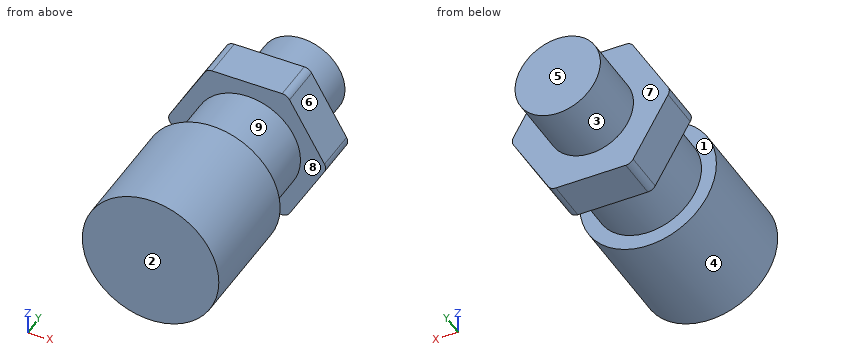
from build123d import *

# Parameters (mm, degrees)
BOSS_EXTRUDE1_DEPTH = 12.7
FILLET1_R           = 2.54
SKETCH2_R           = 20.32
BOSS_EXTRUDE4_DEPTH = 55.626
SKETCH4_R           = 20.32
SKETCH4_R_2         = 15.875
CUT_EXTRUDE1_DEPTH  = 20.32
SKETCH5_R           = 12.7
BOSS_EXTRUDE5_DEPTH = 19.05


with BuildPart() as part:
    # Sketch1 → Boss-Extrude1 (new body)
    with BuildSketch(Plane(origin=(0, 0, 0), x_dir=(1, 0, 0), z_dir=(0, 1, 0))):
        Polygon((-11.878404438, 20.574), (11.878404438, 20.574), (23.756808877, 0), (11.878404438, -20.574), (-11.878404438, -20.574), (-23.756808877, 0), align=None)
    extrude(amount=BOSS_EXTRUDE1_DEPTH)

    # Fillet1
    fillet1_edges = [part.edges().sort_by_distance(p)[0] for p in [
        (-11.878404438, 6.35, -20.574),
        (11.878404438, 6.35, -20.574),
        (23.756808877, 6.35, 0),
        (11.878404438, 6.35, 20.574),
        (-11.878404438, 6.35, 20.574),
        (-23.756808877, 6.35, 0),
    ]]
    fillet(fillet1_edges, radius=FILLET1_R)

    # Sketch2 → Boss-Extrude4 (add)
    with BuildSketch(Plane.XZ):
        Circle(SKETCH2_R)
    extrude(amount=BOSS_EXTRUDE4_DEPTH)

    # Sketch4 → Cut-Extrude1 (cut)
    with BuildSketch(Plane.XZ):
        Circle(SKETCH4_R)
        Circle(SKETCH4_R_2, mode=Mode.SUBTRACT)
    extrude(amount=CUT_EXTRUDE1_DEPTH, mode=Mode.SUBTRACT)

    # Sketch5 → Boss-Extrude5 (add)
    with BuildSketch(Plane(origin=(0, 12.7, 0), x_dir=(1, 0, 0), z_dir=(0, 1, 0))):
        Circle(SKETCH5_R)
    extrude(amount=BOSS_EXTRUDE5_DEPTH)


solid = part.part
Source: CAD feature listing. Evaluate the final solid. Frame: model axes, mm. Face numbers are marked on the shaded views. A direction names the side the tool comes from. Round coordinates to 2 decimals unless told otherwise and drop trailing zeros. Loops run counter-clockwise (first coordinate to the right, second up) from the corner with the lowest first, then second, coordinate; pieces in that order, holes last. Notation, with made-up numbers: (-10.75, 57) -> (10.25, 57) arc R17 ccw to (10.25, 89) -> close; hole circle Ø1 at (16, 77.5). An arc over 180 degrees is marked (long way). Answer as a JSON object with one key per item and string values. Group by question number.
Q1. Ray query, line 1 (Y direction, x = 18, z = -1); line 2 (Y direction, x = -11, z = -18.5); line 3 (Y direction, x = -12.5, z = 9.5). Return the intervals inside material, ascending. Write a range as from..to.
Q2. Mould query, pull axis Y, two halves, no side actions, for the marked faces 6, 7, 8 and 9. Classes: pulls with the +Y half, pulls with the -Y half, needs draft (parallel to the pull), parting line crosses it, or undercut.
Q3. Access query for the marked faces 1, 2, 3, 4 and 5. Directions: +Z, -Z, +X, -X, +Y, -Y. A direction counts if a zero-diameter tool reaches every point of the face in a straight line with its end or side. Return the directions, or none.
Q4. Section query A-A (x = 0). Output: boundary loops of the cut face in (y, z) (3 decimals).
Q5. Section query D-D (z = 0). Output: boundary loops of the cut face in (x, y) (3 decimals).
Q6. Section query C-C (x = -18). Output: boundary loops of the cut face in (y, z).
Q7. Contact query for flat-ended pins moving along their axis: P1, Ø5, axis at x = -5.5, y = -11.5, coming from the -Z side; P2, Ø4, axis at y = 1, z = -2.5, coming from the -X side; P3, Ø1, axis at x = -14.5, z = 6.5, coming from the +Y side. Output: stop coordinate, or through.
Q8. Section query B-B (z = -18). Output: boundary loops of the cut face in (x, y).
Completed:
{
 "1": {"line 1": "-55.63..-20.32, 0..12.7", "line 2": "0..12.7", "line 3": "-55.63..12.7"},
 "2": {"face 6": "needs draft", "face 7": "pulls with the +Y half", "face 8": "undercut", "face 9": "undercut"},
 "3": {"face 1": "none", "face 2": "+Z, -Z, +X, -X, -Y", "face 3": "+Y", "face 4": "-Y", "face 5": "+Z, -Z, +X, -X, +Y"},
 "4": {"outline": "(-55.626, -20.32) -> (-20.32, -20.32) -> (-20.32, -15.875) -> (0, -15.875) -> (0, -20.574) -> (12.7, -20.574) -> (12.7, -12.7) -> (31.75, -12.7) -> (31.75, 12.7) -> (12.7, 12.7) -> (12.7, 20.574) -> (0, 20.574) -> (0, 15.875) -> (-20.32, 15.875) -> (-20.32, 20.32) -> (-55.626, 20.32) -> close"},
 "5": {"outline": "(-23.364, 0) -> (-15.875, 0) -> (-15.875, -20.32) -> (-20.32, -20.32) -> (-20.32, -55.626) -> (20.32, -55.626) -> (20.32, -20.32) -> (15.875, -20.32) -> (15.875, 0) -> (23.364, 0) -> (23.364, 12.7) -> (12.7, 12.7) -> (12.7, 31.75) -> (-12.7, 31.75) -> (-12.7, 12.7) -> (-23.364, 12.7) -> close"},
 "6": {"outline": "(-55.63, -9.43) -> (-20.32, -9.43) -> (-20.32, 9.43) -> (-55.63, 9.43) -> close; (0, -9.97) -> (12.7, -9.97) -> (12.7, 9.97) -> (0, 9.97) -> close"},
 "7": {"P1": "z = -15.59", "P2": "x = -23.31", "P3": "y = 12.7"},
 "8": {"outline": "(-13.36, 0) -> (13.36, 0) -> (13.36, 12.7) -> (-13.36, 12.7) -> close; (-9.43, -55.63) -> (9.43, -55.63) -> (9.43, -20.32) -> (-9.43, -20.32) -> close"}
}
